For this review, use the dimensioned drawing (mm, ordinates from the lowest corner) and the shaded views. Give positions to 0.01 mm unless a question says otherwise; leave off trailing zeros. Loops run counter-clockwise (first coordinate to the right, second up) from the corner with the lowest first, then second, coordinate; pieces in that order, holes last. Notation, with made-up numbers: (68, -5) -> (103, -5) arc R30 cw to (103, 17) -> close; hole circle Ø5 at (78.25, 41). An arc over 180 degrees is marked (long way). Use a Markdown table: item, result. Add a question column.
1. Add section A-A (z = 9.5). State the section outline as (x, y) points, and give its area (3 significant figures).
2. Add section D-D (x = 15.5). State the section outline as (y, z) points, and give its area (3 significant figures).
3. To check wall thickness, follow line 1 (Z direction, x = 14.5, y = 4.75); line 2 (Z direction, x = 4.75, y = 7.75); line 3 (X direction, y = 8.25, z = 11.25). State the ranges of each line that lie inside material, in increasing order.
4. Draft analysis for pull direction X (two halves, no side actions). For the marked faces 1, 2 and 3, state which applies: pulls with the +X half, pulls with the -X half, needs draft (parallel to the pull), parting line crosses it, or undercut.
5. Add section B-B (x = 5.75). State the section outline as (y, z) points.
6. For pin 1 Ø6 at (y, z) = (2, 4) entering from +X; pin 2 Ø5 at (y, z) = (4.5, 7.5) entering from +X; pin 3 Ø4 at (x, y) = (14.5, 1) entering from -Z; pin 4 Ø2 at (y, z) = (4.5, 13) entering from -X, all flat-tipped, find the tip position at first contact; note any pin that passes through.
7. Add section C-C (y = 4). State the section outline as (x, z) points.
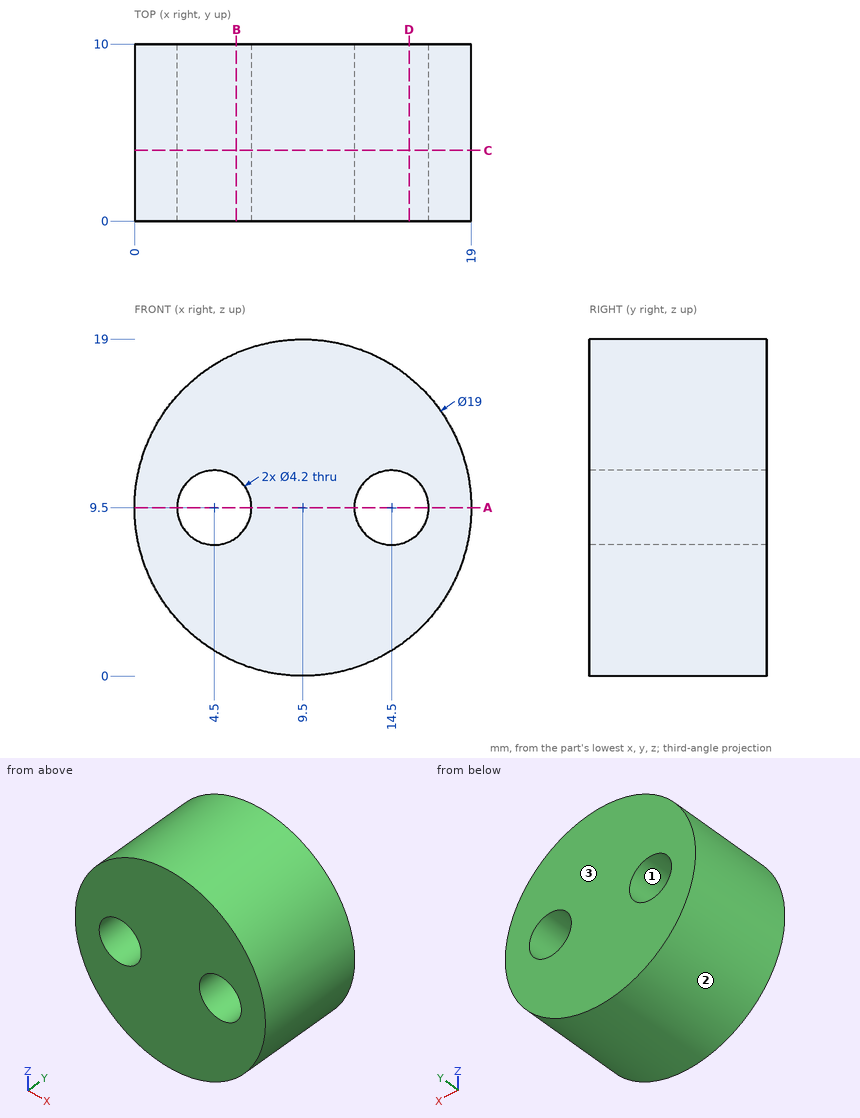
Taken from the geometry:
| question | item | result |
|---|---|---|
| 1 | outline | (0, 0) -> (2.4, 0) -> (2.4, 10) -> (0, 10) -> close; (6.6, 0) -> (12.4, 0) -> (12.4, 10) -> (6.6, 10) -> close; (16.6, 0) -> (19, 0) -> (19, 10) -> (16.6, 10) -> close |
| 1 | area | 106 mm^2 |
| 2 | outline | (0, 2.13) -> (10, 2.13) -> (10, 7.65) -> (0, 7.65) -> close; (0, 11.35) -> (10, 11.35) -> (10, 16.87) -> (0, 16.87) -> close |
| 2 | area | 110 mm^2 |
| 3 | line 1 | z = 1.42 to 7.4, 11.6 to 17.58 |
| 3 | line 2 | z = 1.27 to 7.41, 11.59 to 17.73 |
| 3 | line 3 | x = 0.16 to 3.34, 5.66 to 13.34, 15.66 to 18.84 |
| 4 | face 1 | undercut |
| 4 | face 2 | parting line crosses it |
| 4 | face 3 | needs draft |
| 5 | outline | (0, 0.77) -> (10, 0.77) -> (10, 7.81) -> (0, 7.81) -> close; (0, 11.19) -> (10, 11.19) -> (10, 18.23) -> (0, 18.23) -> close |
| 6 | pin 1 | stops at x = 18.67 |
| 6 | pin 2 | stops at x = 19 |
| 6 | pin 3 | stops at z = 0.49 |
| 6 | pin 4 | stops at x = 0.33 |
| 7 | outline | circle Ø19 at (9.5, 9.5); hole circle Ø4.2 at (4.5, 9.5); hole circle Ø4.2 at (14.5, 9.5) |
